Input: part model. Units: mm. Frame: model coordinates. Give positions to 0.01 mm unless a question says otherwise; leave off trailing zeros. Order: outer loops, then holes, each group sorted by start corner. A loop starts at its lowest first (then second) coordinate and runs counter-clockwise, first axis right, second up. Notation, with made-up numbers: M 45.25,53.5 L 87.25,53.5 A33 cw 87.25,86.5 Z; hole C 36,-18.5 d5. An arc over 180 degrees is marked long. Use a Markdown table: item, result.
from build123d import *

# Parameters (mm, degrees)
F1_DEPTH = 3.048


with BuildPart() as f1:
    # F0 (on Front) → F1 (new body)
    with BuildSketch(Plane.XZ):
        with BuildLine():
            Line((0, 28.1219437212), (0, 33.5548328109))
            ThreePointArc((0, 33.5548328109), (-7.0011965198, 36.6215921611), (-9.4940497557, 43.8470643509))
            Line((-9.4940497557, 43.8470643509), (-14.5120441123, 6.4355419883))
            ThreePointArc((-14.5120441123, 6.4355419883), (-8.655963145, 13.3075139313), (0, 15.875))
            Line((0, 15.875), (0, 24.9469437212))
            ThreePointArc((0, 24.9469437212), (-1.5875, 26.5344437212), (0, 28.1219437212))
        make_face()
        with BuildLine():
            ThreePointArc((-9.4940497557, 43.8470643509), (-7.0011965198, 36.6215921611), (0, 33.5548328109))
            ThreePointArc((0, 33.5548328109), (6.055219513, 35.7272862011), (9.3483010398, 41.2536639606))
            ThreePointArc((9.3483010398, 41.2536639606), (9.480722346, 42.1624840233), (9.525, 43.0798328109))
            ThreePointArc((9.525, 43.0798328109), (0.3839277776, 52.5970921045), (-9.4940497557, 43.8470643509))
        make_face()
        with BuildLine():
            ThreePointArc((1.5875, 43.0798328109), (1.1225320151, 41.9573007958), (0, 41.4923328109))
            ThreePointArc((0, 41.4923328109), (-1.1225320151, 44.2023648261), (1.5875, 43.0798328109))
        make_face(mode=Mode.SUBTRACT)
        with BuildLine():
            ThreePointArc((9.3483010398, 41.2536639606), (6.055219513, 35.7272862011), (0, 33.5548328109))
            Line((0, 33.5548328109), (0, 28.1219437212))
            ThreePointArc((0, 28.1219437212), (1.1225320151, 27.6569757363), (1.5875, 26.5344437212))
            ThreePointArc((1.5875, 26.5344437212), (1.1225320151, 25.411911706), (0, 24.9469437212))
            Line((0, 24.9469437212), (0, 15.875))
            ThreePointArc((0, 15.875), (10.2809992556, 12.0961431583), (15.6674568575, 2.558597393))
            Line((15.6674568575, 2.558597393), (9.3483010398, 41.2536639606))
        make_face()
        with BuildLine():
            ThreePointArc((15.875, 0), (15.8230291445, 1.2835005625), (15.6674568575, 2.558597393))
            ThreePointArc((15.6674568575, 2.558597393), (10.2809992556, 12.0961431583), (0, 15.875))
            Line((0, 15.875), (0, 3.175))
            ThreePointArc((0, 3.175), (2.2450640303, 2.2450640303), (3.175, 0))
            ThreePointArc((3.175, 0), (2.2450640303, -2.2450640303), (0, -3.175))
            Line((0, -3.175), (0, -15.875))
            ThreePointArc((0, -15.875), (9.5773172553, -12.6605931611), (15.2761596654, -4.3190937564))
            ThreePointArc((15.2761596654, -4.3190937564), (15.7245772549, -2.1802053013), (15.875, 0))
        make_face()
        with BuildLine():
            ThreePointArc((0, 15.875), (-8.655963145, 13.3075139313), (-14.5120441123, 6.4355419883))
            Line((-14.5120441123, 6.4355419883), (-15.6949904948, -2.3838830444))
            ThreePointArc((-15.6949904948, -2.3838830444), (-15.3752760195, -3.951773314), (-14.8993476116, -5.4795132768))
            ThreePointArc((-14.8993476116, -5.4795132768), (-9.0837313845, -13.0192722198), (0, -15.875))
            Line((0, -15.875), (0, -3.175))
            ThreePointArc((0, -3.175), (-3.175, 0), (0, 3.175))
            Line((0, 3.175), (0, 15.875))
        make_face()
        with BuildLine():
            ThreePointArc((0, -15.875), (-9.0837313845, -13.0192722198), (-14.8993476116, -5.4795132768))
            Line((-14.8993476116, -5.4795132768), (-9.4394359543, -45.9385966374))
            ThreePointArc((-9.4394359543, -45.9385966374), (-7.1714354085, -38.3960912017), (0, -35.1397544709))
            Line((0, -35.1397544709), (0, -15.875))
        make_face()
        with BuildLine():
            Line((10.6975523741, -36.9681615729), (15.2761596654, -4.3190937564))
            ThreePointArc((15.2761596654, -4.3190937564), (9.5773172553, -12.6605931611), (0, -15.875))
            Line((0, -15.875), (0, -35.1397544709))
            ThreePointArc((0, -35.1397544709), (2.9798902503, -35.6178832384), (5.660615933, -37.0042680464))
            Line((5.660615933, -37.0042680464), (10.6975523741, -36.9681615729))
        make_face()
        with BuildLine():
            ThreePointArc((5.660615933, -37.0042680464), (2.9798902503, -35.6178832384), (0, -35.1397544709))
            Line((0, -35.1397544709), (0, -43.0772544709))
            ThreePointArc((0, -43.0772544709), (1.1225320151, -43.5422224557), (1.5875, -44.6647544709))
            Line((1.5875, -44.6647544709), (9.525, -44.6647544709))
            ThreePointArc((9.525, -44.6647544709), (8.5042046001, -40.374751077), (5.660615933, -37.0042680464))
        make_face()
        with BuildLine():
            ThreePointArc((0, -35.1397544709), (-7.1714354085, -38.3960912017), (-9.4394359543, -45.9385966374))
            ThreePointArc((-9.4394359543, -45.9385966374), (-6.2686632691, -51.8361898794), (0, -54.1897544709))
            Line((0, -54.1897544709), (0.6791137982, -54.1655138852))
            ThreePointArc((0.6791137982, -54.1655138852), (6.9711614501, -51.155404133), (9.525, -44.6647544709))
            Line((9.525, -44.6647544709), (1.5875, -44.6647544709))
            ThreePointArc((1.5875, -44.6647544709), (-1.1225320151, -45.787286486), (0, -43.0772544709))
            Line((0, -43.0772544709), (0, -35.1397544709))
        make_face()
        with BuildLine():
            Line((9.6182052834, -44.6647544709), (10.6975523741, -36.9681615729))
            Line((10.6975523741, -36.9681615729), (5.660615933, -37.0042680464))
            ThreePointArc((5.660615933, -37.0042680464), (8.5042046001, -40.374751077), (9.525, -44.6647544709))
            Line((9.525, -44.6647544709), (9.6182052834, -44.6647544709))
        make_face()
        with BuildLine():
            Line((44.2762012087, -36.7274583976), (10.6975523741, -36.9681615729))
            Line((10.6975523741, -36.9681615729), (9.6182052834, -44.6647544709))
            Line((9.6182052834, -44.6647544709), (36.3955984465, -44.6647544709))
            ThreePointArc((36.3955984465, -44.6647544709), (38.7003580799, -39.0722467854), (44.2762012087, -36.7274583976))
        make_face()
        with BuildLine():
            Line((36.3955984465, -44.6647544709), (9.6182052834, -44.6647544709))
            Line((9.6182052834, -44.6647544709), (9.525, -44.6647544709))
            ThreePointArc((9.525, -44.6647544709), (6.9711614501, -51.155404133), (0.6791137982, -54.1655138852))
            Line((0.6791137982, -54.1655138852), (44.6162427329, -52.5972027413))
            ThreePointArc((44.6162427329, -52.5972027413), (38.8214540242, -50.3766440016), (36.3955984465, -44.6647544709))
        make_face()
        with BuildLine():
            ThreePointArc((52.2705984465, -44.6647544709), (49.925606132, -39.0320141043), (44.2762012087, -36.7274583976))
            ThreePointArc((44.2762012087, -36.7274583976), (38.7003580799, -39.0722467854), (36.3955984465, -44.6647544709))
            ThreePointArc((36.3955984465, -44.6647544709), (38.8214540242, -50.3766440016), (44.6162427329, -52.5972027413))
            ThreePointArc((44.6162427329, -52.5972027413), (50.0449879773, -50.1763988932), (52.2705984465, -44.6647544709))
        make_face()
        with BuildLine():
            ThreePointArc((45.9205984465, -44.6647544709), (44.3330984465, -46.2522544709), (42.7455984465, -44.6647544709))
            ThreePointArc((42.7455984465, -44.6647544709), (44.3330984465, -43.0772544709), (45.9205984465, -44.6647544709))
        make_face(mode=Mode.SUBTRACT)
    extrude(amount=F1_DEPTH)


solid = f1.part
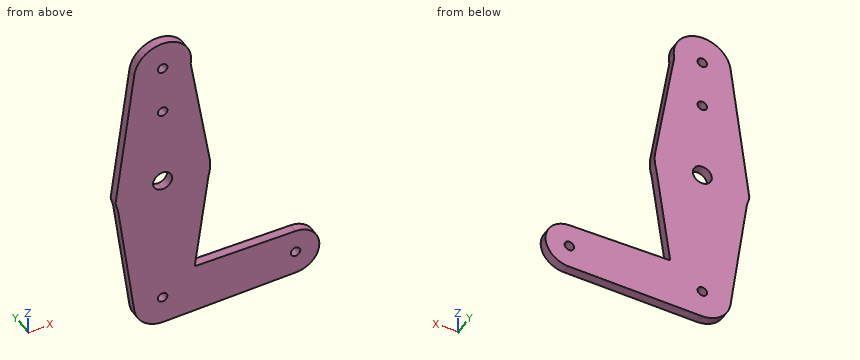
1) Cut plane B-B on z = 35. Return loops of the section in (x, y), and give its area (3 significant figures).
Response values:
| item | result |
|---|---|
| outline | M -10.68,-3.05 L 10.37,-3.05 L 10.37,0 L -10.68,0 Z |
| area | 64.2 mm² |
2) Cut plane C-C on x = 48.5. Return loops of the section in (y, z), and give its area (3 significant figures).
Response values:
| item | result |
|---|---|
| outline | M -3.05,-51.42 L 0,-51.42 L 0,-37.91 L -3.05,-37.91 Z |
| area | 41.2 mm² |
3) Material intervals for line 1 (Z direction, x = -1, y = -2.5); line 2 (X direction, y = -0.35, z = 12); line 3 (X direction, y = -1.8, z = 44.5), sorted ascending. Write a range as from..to.
Response values:
| item | result |
|---|---|
| line 1 | z = -54.14..-45.9, -43.43..-3.01, 3.01..25.3, 27.77..41.85, 44.31..52.55 |
| line 2 | x = -13.77..14.13 |
| line 3 | x = -9.42..-0.71, 0.71..9.42 |
4) Cut plane A-A on y = -2.5. State how many separate pieces and enclosed holes the cut face has, and give its area (3 significant figures).
Response values:
| item | result |
|---|---|
| separate pieces | 1 |
| enclosed holes | 5 |
| area | 3,120 mm² |
